```python
from build123d import *

# Parameters (mm, degrees)
SKETCH_1_R      = 1
EXTRUDE_1_DEPTH = 3
FILLET_1_R      = 3.81


with BuildPart() as part:
    # 스케치1 → 보스-돌출1 (new body)
    with BuildSketch(Plane.XY):
        with BuildLine():
            ThreePointArc((1.360143251, -0.016380398), (7.940783027, -1.841517038), (1.212921566, -3.01276585))
            ThreePointArc((1.212921566, -3.01276585), (0, -2.999009296), (-1.212921566, -3.01276585))
            ThreePointArc((-1.212921566, -3.01276585), (-7.940783027, -1.841517038), (-1.360143251, -0.016380398))
            ThreePointArc((-1.360143251, -0.016380398), (0, 0), (1.360143251, -0.016380398))
        make_face()
        with Locations((-4.445, -1.669758406)):
            Circle(SKETCH_1_R, mode=Mode.SUBTRACT)
        with Locations((4.445, -1.669758406)):
            Circle(SKETCH_1_R, mode=Mode.SUBTRACT)
    extrude(amount=EXTRUDE_1_DEPTH)

    # 필렛1
    # the kernel refuses this fillet: 3.81 mm, written as the material it adds along each edge
    with BuildSketch(Plane(origin=(1.212921566, -3.01276585, 0), x_dir=(0.5541029817307234, -0.8324481278957396, 0), z_dir=(0, 0, 1))) as fillet_1_piece_1:
        with BuildLine():
            CenterArc((2.078362303, -3.73891854), FILLET_1_R, 101.084875911, 46.128957788)
            ThreePointArc((-1.12469468, -1.675783557), (-0.570253257, -0.832585758), (0, 0))
            ThreePointArc((0, 0), (0.672920265, -0.065297929), (1.345840529, 0))
        make_face()
    extrude(amount=3)
    with BuildSketch(Plane(origin=(-1.212921566, -3.01276585, 0), x_dir=(-0.5541029817307197, -0.8324481278957422, 0), z_dir=(0, 0, 1))) as fillet_1_piece_2:
        with BuildLine():
            CenterArc((2.078362303, 3.73891854), FILLET_1_R, 212.786166302, 46.128957788)
            ThreePointArc((-1.12469468, 1.675783557), (-0.570253257, 0.832585758), (0, 0))
            ThreePointArc((0, 0), (0.672920265, 0.065297929), (1.345840529, 0))
        make_face()
    extrude(amount=3)
    with BuildSketch(Plane(origin=(1.360143251, -0.016380398, 0), x_dir=(-0.9999615504987989, 0.008769123333507087, 0), z_dir=(0, 0, 1))) as fillet_1_piece_3:
        with BuildLine():
            CenterArc((1.788298707, -3.809553141), FILLET_1_R, 90.877535516, 41.082301134)
            ThreePointArc((-0.759103528, -0.976384975), (-0.336083058, -0.521987813), (0, 0))
            ThreePointArc((0, 0), (0.864973735, -0.006624048), (1.72994747, 0))
        make_face()
    extrude(amount=3)
    with BuildSketch(Plane(origin=(-1.360143251, -0.016380398, 0), x_dir=(-0.6206853131175095, 0.7840597822106544, 0), z_dir=(0, 0, 1))) as fillet_1_piece_4:
        with BuildLine():
            CenterArc((1.909904861, -3.750062775), FILLET_1_R, 100.176406591, 41.082301134)
            ThreePointArc((-1.061817419, -1.365745957), (-0.525679205, -0.686938726), (0, 0))
            ThreePointArc((0, 0), (0.618378077, -0.055060443), (1.236756154, 0))
        make_face()
    extrude(amount=3)


solid = part.part
```
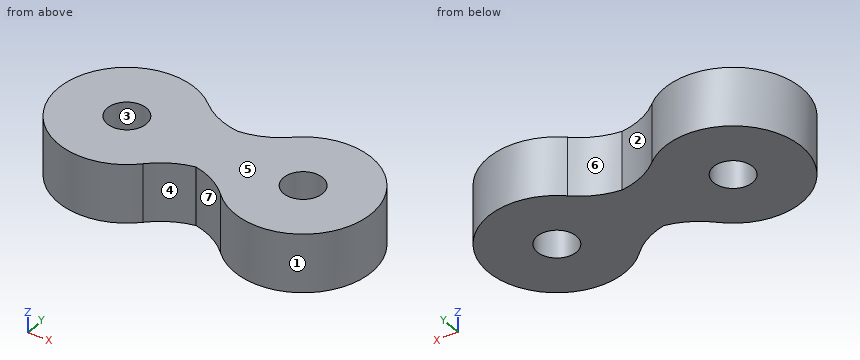
Geometry: final body of the model. Coordinates: model frame, mm. Face numbers are marked on the shaded views. A direction names the side the tool comes from. Round coordinates to 2 decimals unless told otherwise and drop trailing zeros. Write each loop counter-clockwise with the first axis right and the second up, starting at its lowest first coordinate (ties: lowest second). Pieces come first, ordered by that corner, then holes. Notation, with made-up numbers: (14.5, 12) -> (19.5, 12) arc R9 cw to (19.5, 26) -> close; hole circle Ø6 at (44.5, 72). An arc over 180 degrees is marked (long way). Use CSV: the item, a comma, the result in double quotes. Start each with the question number.
Q1. Pull-direction query (Y, two-part tool) for the marked faces 1, 2, 3 and 4; classes: pulls with the +Y half, pulls with the -Y half, needs draft (parallel to the pull), parting line crosses it, or undercut.
Q2. Section B-B (z = 1.15). Return loops of the section in (x, y) (3 decimals).
Q3. Reachability of the marked faces 5, 6 and 7 from +Z, -Z, +X, -X, +Y, -Y: full face, straight path, thin tool, end or side. Return the list, or none.
Q4. First-contact query: pin 1 Ø1.5 at (x, z) = (1.5, 0.5) entering from -Y. Flat tip, straight axial feed; report the tip coordinate or a pass-through.
Q5. Section C-C (x = -5). Return loops of the section in (y, z), plus the area to 3 significant figures.
Q6. Line query: L1, parallel to X at y = -1.5, z = 1.05; L2, parallel to Y at x = -4.5, z = 2.2; L3, parallel to X at y = 0.5, z = 2.8. Output: solid intervals per line, ascending.
Q7. Section A-A (y = 1.25). Return loops of the section in (x, z), plus the area to 3 significant figures.
Q8. Section D-D (y = -2.5). Return loops of the section in (x, z).
Result sheet:
1,face 1,"parting line crosses it"
1,face 2,"pulls with the +Y half"
1,face 3,"undercut"
1,face 4,"pulls with the -Y half"
2,outline,"(-2.128, 0.953) arc R3.5 ccw (long way) to (-1.959, -4.133) arc R3.81 cw to (0, -3.079) arc R3.81 cw to (1.959, -4.133) arc R3.5 ccw (long way) to (2.128, 0.953) arc R3.81 cw to (0, 0.019) arc R3.81 cw to start; hole circle Ø2 at (-4.445, -1.67); hole circle Ø2 at (4.445, -1.67)"
3,face 5,"+Z, +X, -X, +Y, -Y"
3,face 6,"+Z, -Z, +Y"
3,face 7,"+Z, -Z, -Y"
4,pin 1,"y = -4.4"
5,outline,"(-5.13, 0) -> (-2.5, 0) -> (-2.5, 3) -> (-5.13, 3) -> close; (-0.84, 0) -> (1.79, 0) -> (1.79, 3) -> (-0.84, 3) -> close"
5,area,"15.7 mm²"
6,L1,"-7.94 to -5.43, -3.46 to 3.46, 5.43 to 7.94"
6,L2,"-5.17 to -2.67, -0.67 to 1.83"
6,L3,"-7.19 to -1.49, 1.49 to 7.19"
7,outline,"(-6.38, 0) -> (-2.51, 0) -> (-2.51, 3) -> (-6.38, 3) -> close; (2.51, 0) -> (6.38, 0) -> (6.38, 3) -> (2.51, 3) -> close"
7,area,"23.2 mm²"
8,outline,"(-7.85, 0) -> (-5, 0) -> (-5, 3) -> (-7.85, 3) -> close; (-3.89, 0) -> (3.89, 0) -> (3.89, 3) -> (-3.89, 3) -> close; (5, 0) -> (7.85, 0) -> (7.85, 3) -> (5, 3) -> close"
